Design review of the part shown in the three views and the two pictorial views. Dimensions are in mm from the part's minimum x, y and z. A direction names the side the tool comes from. Coordinates: 2 decimals unless noted, no trailing zeros. Loops run counter-clockwise (first coordinate to the right, second up) from the corner with the lowest first, then second, coordinate; pieces in that order, holes last. Notation, with made-up numbers: (-27, 72) -> (13, 72) arc R16 ccw to (13, 88) -> close; hole circle Ø2 at (32.25, 2). An arc over 180 degrees is marked (long way). Answer in a Markdown table with one row per item.
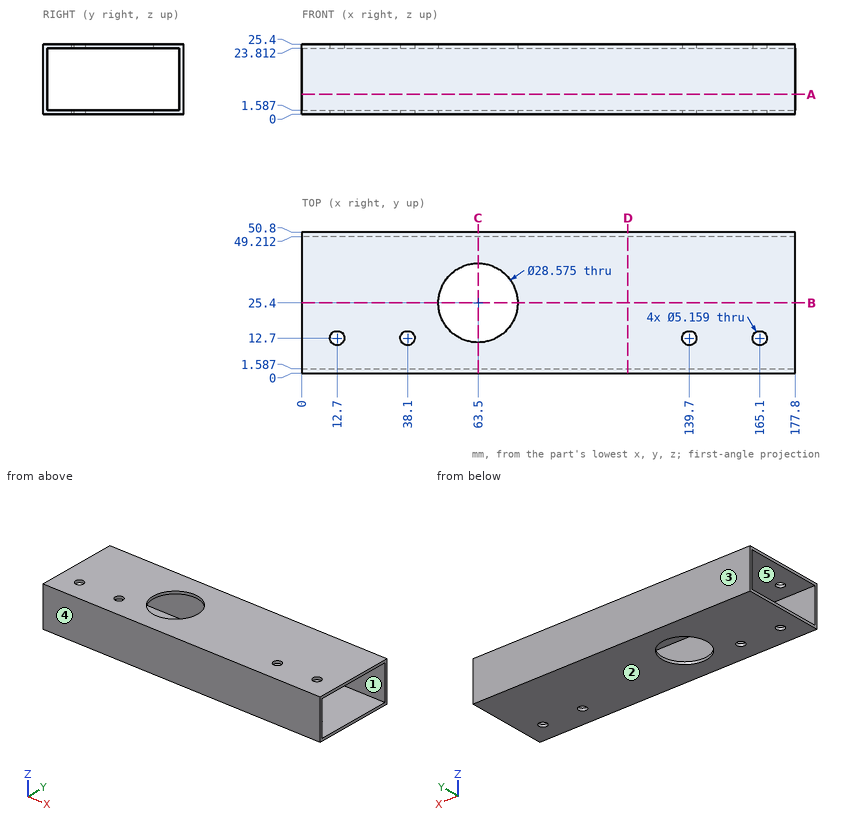
Item 1: For the marked faces 4 and 5, list the 3-axis set-ups (+Z, -Z, +X, -X, +Y, -Y) from which the entire face can be reached by the end or side of a thin tool; tool diameter is ignored.
Worked answers:
| item | result |
|---|---|
| face 4 | +Z, -Z, +X, -X, -Y |
| face 5 | +X, -X |
Item 2: Take a section at B-B, the plane y = 25.4. State the section outline as (x, z) points.
Worked answers:
| item | result |
|---|---|
| outline | (0, 0) -> (49.21, 0) -> (49.21, 1.59) -> (0, 1.59) -> close; (0, 23.81) -> (49.21, 23.81) -> (49.21, 25.4) -> (0, 25.4) -> close; (77.79, 0) -> (177.8, 0) -> (177.8, 1.59) -> (77.79, 1.59) -> close; (77.79, 23.81) -> (177.8, 23.81) -> (177.8, 25.4) -> (77.79, 25.4) -> close |
Item 3: Take a section at C-C, the plane x = 63.5. State the section outline as (y, z) points.
Worked answers:
| item | result |
|---|---|
| outline | (0, 0) -> (11.11, 0) -> (11.11, 1.59) -> (1.59, 1.59) -> (1.59, 23.81) -> (11.11, 23.81) -> (11.11, 25.4) -> (0, 25.4) -> close; (39.69, 0) -> (50.8, 0) -> (50.8, 25.4) -> (39.69, 25.4) -> (39.69, 23.81) -> (49.21, 23.81) -> (49.21, 1.59) -> (39.69, 1.59) -> close |
Item 4: Take a section at A-A, the plane z = 7.25. State the section outline as (x, y) points.
Worked answers:
| item | result |
|---|---|
| outline | (0, 0) -> (177.8, 0) -> (177.8, 1.59) -> (0, 1.59) -> close; (0, 49.21) -> (177.8, 49.21) -> (177.8, 50.8) -> (0, 50.8) -> close |
Item 5: The part is to be moulded in two halves that separate along Y. For the marked faces 1, 2 and 3, say which applies: +Y half, -Y half, draft (parallel to the pull), parting line (faces both ways), or undercut.
Worked answers:
| item | result |
|---|---|
| face 1 | undercut |
| face 2 | draft |
| face 3 | +Y half |
Item 6: Take a section at D-D, the plane x = 117.5. State the section outline as (y, z) points, and give its area (3 significant figures).
Worked answers:
| item | result |
|---|---|
| outline | (0, 0) -> (50.8, 0) -> (50.8, 25.4) -> (0, 25.4) -> close; hole (1.59, 1.59) -> (49.21, 1.59) -> (49.21, 23.81) -> (1.59, 23.81) -> close |
| area | 232 mm² |
Item 7: For L1, parallel to Z at x = 86.5, y = 12; L2, parallel to Y at x = 38.1, z = 24.55; L3, parallel to Y at x = 169, z = 20, list the stretches that pass through material, from the lowest coordinate up.
Worked answers:
| item | result |
|---|---|
| L1 | 0 to 1.59, 23.81 to 25.4 |
| L2 | 0 to 10.12, 15.28 to 50.8 |
| L3 | 0 to 1.59, 49.21 to 50.8 |
